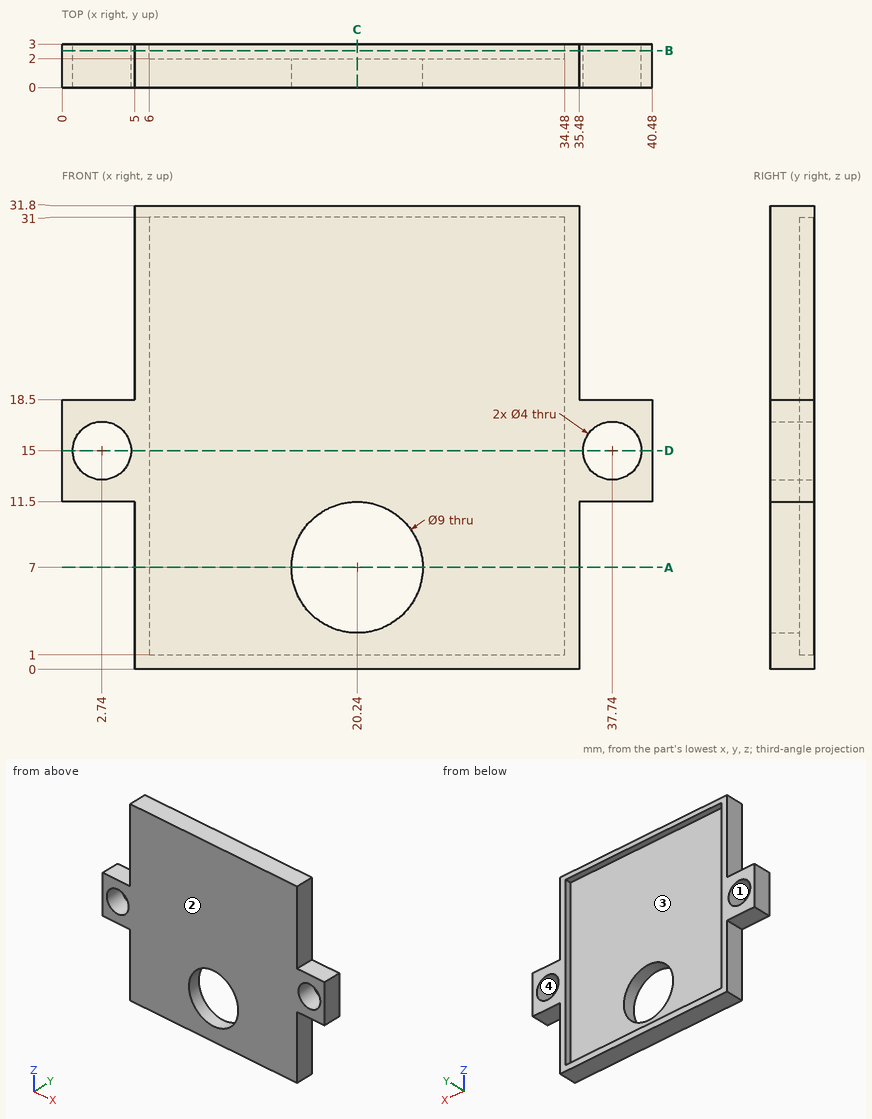
For this review, use the dimensioned drawing (mm, ordinates from the lowest corner) and the shaded views. A direction names the side the tool comes from. Give positions to 0.01 mm unless a question says otherwise; leave off trailing zeros. Loops run counter-clockwise (first coordinate to the right, second up) from the corner with the lowest first, then second, coordinate; pieces in that order, holes last.
Item 1: Take a section at C-C, the plane x = 20.24. State the section outline as (y, z) points, and give its area (3 significant figures).
Item 2: Draft analysis for pull direction X (two halves, no side actions). For the marked faces 1 and 2, state which applies: +X half, -X half, draft (parallel to the pull), parting line (faces both ways), or undercut.
Item 3: Take a section at A-A, the plane z = 7. State the section outline as (x, y) points, and give its area (3 significant figures).
Item 4: Tool access review of the marked faces 3 and 4: name each direction out of +Z, -Z, +X, -X, +Y, -Y from which nothing blocks a thin tool from reaching the whole face with its end or side.
Item 5: Insertion check: pin 1 (4 mm diameter, centred on x = 23, z = 26, fed in from +Y); pin 2 (0.9 mm diameter, centred on y = 1.5, z = 7, fed in from +X); pin 3 (1.5 mm diameter, centred on x = 38, y = 2, fed in from +Z). Each pin has a flat end and moves straight along its axis. Give the tip position at first contact, or say it passes through.
Item 6: Take a section at B-B, the plane y = 2.55. State the section outline as (x, z) points.
Item 7: For line 1 along Z through (x, y) = (37.74, 0.85); line 2 along Z through (x, y) = (20.24, 1.2); line 3 along X through (y, z) = (2.9, 15.5), list the stretches that pass through material, from the lowest coordinate up.
Item 8: Take a section at D-D, the plane z = 15. State the section outline as (x, y) points, and give its area (3 significant figures).
Calculated:
1. outline: (0, 0) - (3, 0) - (3, 1) - (2, 1) - (2, 2.5) - (0, 2.5) - close; (0, 11.5) - (2, 11.5) - (2, 31) - (3, 31) - (3, 31.8) - (0, 31.8) - close
1. area: 47.4 mm2
2. face 1: undercut
2. face 2: draft
3. outline: (5, 0) - (15.74, 0) - (15.74, 2) - (6, 2) - (6, 3) - (5, 3) - close; (24.74, 0) - (35.48, 0) - (35.48, 3) - (34.48, 3) - (34.48, 2) - (24.74, 2) - close
3. area: 45.0 mm2
4. face 3: +Y
4. face 4: +Y, -Y
5. pin 1: stops at y = 2
5. pin 2: stops at x = 35.48
5. pin 3: stops at z = 18.5
6. outline: (0, 11.5) - (5, 11.5) - (5, 0) - (35.48, 0) - (35.48, 11.5) - (40.48, 11.5) - (40.48, 18.5) - (35.48, 18.5) - (35.48, 31.8) - (5, 31.8) - (5, 18.5) - (0, 18.5) - close; hole circle Ø4 at (2.74, 15); hole (6, 1) - (34.48, 1) - (34.48, 31) - (6, 31) - close; hole circle Ø4 at (37.74, 15)
7. line 1: z = 11.5 to 13, 17 to 18.5
7. line 2: z = 0 to 2.5, 11.5 to 31.8
7. line 3: x = 0 to 0.8, 4.68 to 6, 34.48 to 35.8, 39.68 to 40.48
8. outline: (0, 0) - (0.74, 0) - (0.74, 3) - (0, 3) - close; (4.74, 0) - (35.74, 0) - (35.74, 3) - (34.48, 3) - (34.48, 2) - (6, 2) - (6, 3) - (4.74, 3) - close; (39.74, 0) - (40.48, 0) - (40.48, 3) - (39.74, 3) - close
8. area: 69.0 mm2
